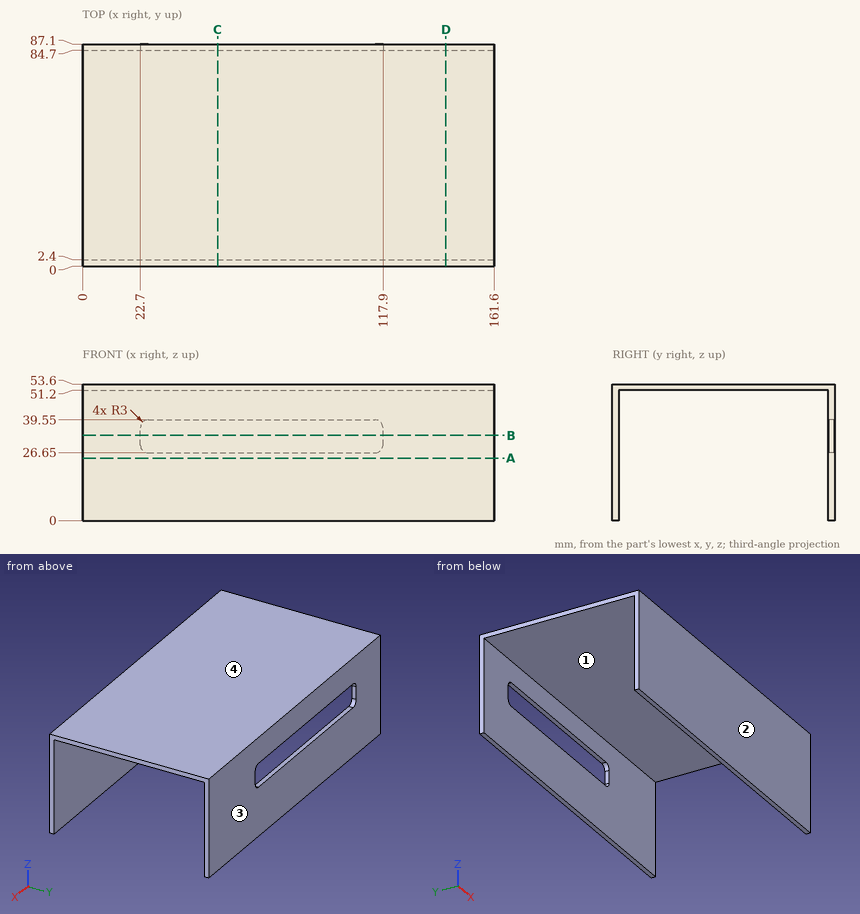
Input: dimensioned drawing with shaded views. Units: mm. Origin: part minimum x, y, z. Give positions to 0.01 mm unless a question says otherwise; leave off trailing zeros. Order: outer loops, then holes, each group sorted by start corner. A loop starts at its lowest first (then second) coordinate and runs counter-clockwise, first axis right, second up. Notation, with made-up numbers: (-38.75, -32.5) -> (-18.75, -32.5) arc R27 ccw to (-18.75, 0.5) -> close; hole circle Ø2 at (9, 14.25). An arc over 180 degrees is marked (long way). Answer as a JSON object with one key per item and string values.
Q1. First-contact query: pin 1 (12 mm diameter, centred on x = 22, y = 10.5, fed in from -Z). Flat tip, straight axial feed; report the tip coordinate or a pass-through.
Entries:
{"pin 1": "stops at z = 51.2"}
Q2. Section C-C (x = 53). Output: boundary loops of the cut face in (y, z).
Entries:
{"outline": "(0, 0) -> (2.4, 0) -> (2.4, 51.2) -> (84.7, 51.2) -> (84.7, 39.55) -> (87.1, 39.55) -> (87.1, 53.6) -> (0, 53.6) -> close; (84.7, 0) -> (87.1, 0) -> (87.1, 26.65) -> (84.7, 26.65) -> close"}
Q3. Section D-D (x = 142.5). Output: boundary loops of the cut face in (y, z), plus the area to 3 significant figures.
Entries:
{"outline": "(0, 0) -> (2.4, 0) -> (2.4, 51.2) -> (84.7, 51.2) -> (84.7, 0) -> (87.1, 0) -> (87.1, 53.6) -> (0, 53.6) -> close", "area": "455 mm^2"}
Q4. Section B-B (z = 33.5). Output: boundary loops of the cut face in (x, y).
Entries:
{"outline": "(0, 0) -> (161.6, 0) -> (161.6, 2.4) -> (0, 2.4) -> close; (0, 84.7) -> (22.7, 84.7) -> (22.7, 87.1) -> (0, 87.1) -> close; (117.9, 84.7) -> (161.6, 84.7) -> (161.6, 87.1) -> (117.9, 87.1) -> close"}
Q5. Section A-A (z = 24.5). Output: boundary loops of the cut face in (x, y).
Entries:
{"outline": "(0, 0) -> (161.6, 0) -> (161.6, 2.4) -> (0, 2.4) -> close; (0, 84.7) -> (161.6, 84.7) -> (161.6, 87.1) -> (0, 87.1) -> close"}
Q6. Material intervals for probe 1 along Y at (x, z) = (112.5, 51); probe 2 along Z at (x, y) = (91.5, 79); probe 3 along Y at (x, z) = (102, 31), sorted ascending.
Entries:
{"probe 1": "y = 0 to 2.4, 84.7 to 87.1", "probe 2": "z = 51.2 to 53.6", "probe 3": "y = 0 to 2.4"}
Q7. Draft query along Y for the marked faces 1, 2, 3 and 4. Return one class per face: released by +Y, released by -Y, zero draft, split by the parting line, or undercut.
Entries:
{"face 1": "undercut", "face 2": "released by -Y", "face 3": "released by +Y", "face 4": "zero draft"}
